Work out the finished part from the listing and answer in its coordinate system (mm). Face numbers are marked on the shaded views. A direction names the side the tool comes from. Coordinates: 2 decimals unless noted, no trailing zeros. Order: outer loops, then holes, each group sorted by start corner. A loop starts at its lowest first (then second) coordinate and runs counter-clockwise, first axis right, second up.
1. Flat-ended cylindrical pins translate along their axes: pin 1 Ø3 at (x, y) = (17.5, -11) entering from +Z; pin 2 Ø6 at (x, z) = (17.5, 7.5) entering from -Y; pin 3 Ø1.1 at (x, z) = (7.5, -3.5) entering from +Y. Find the tip coordinate at first contact, or state that the pin passes through.
2. The part is cut by section C-C, the plane z = 0. Give the vertices of the cut face in (x, y).
3. The part is cut by section D-D, the plane x = 14.5. Give the vertices of the cut face in (y, z).
4. Find the intervals of material crossed by probe 1 along X at (y, z) = (1, 14); probe 2 along Z at (x, y) = (-10, -18); probe 3 along Z at (x, y) = (7.5, -10), in increasing order.
5. The part is cut by section B-B, the plane y = -8. Give the vertices of the cut face in (x, z).
6. Determine the mould class of the marked faces 5, 6 and 7 for opening direction X: +X half, -X half, draft (parallel to the pull), parting line (faces both ways), or undercut.
7. A tool of negligible diameter and unlimited length cuts with its end or side. For the marked faces 1, 2, 3 and 4, from which of +Z, -Z, +X, -X, +Y, -Y can it reach the whole face along a straight path? Write none if from no direction.
8. The part is cut by section A-A, the plane z = -14. Give the vertices of the cut face in (x, y).
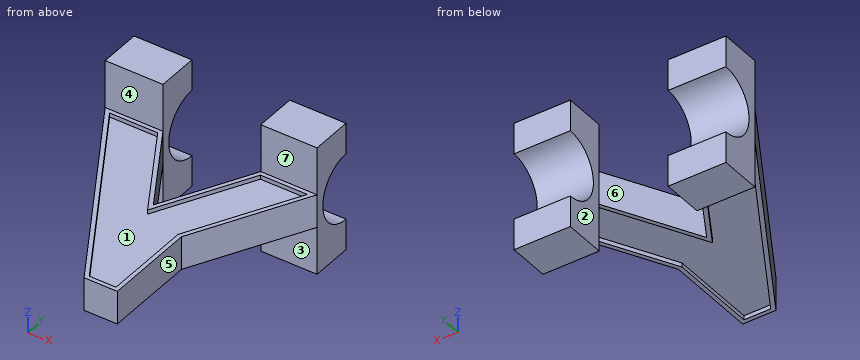
```python
from build123d import *

# Parameters (mm, degrees)
SKETCH_1_W          = 51
SKETCH_1_H          = 31
EXTRUDE_1_DEPTH     = 10
SKETCH_2_R          = 8
CUT_EXTRUDE_1_DEPTH = 51
SKETCH_3_W          = 51
SKETCH_3_H          = 8
EXTRUDE_3_DEPTH     = 49
CUT_EXTRUDE_4_DEPTH = 49
CUT_EXTRUDE_5_DEPTH = 49
CUT_EXTRUDE_6_DEPTH = 1
CUT_EXTRUDE_7_DEPTH = 1


with BuildPart() as part:
    # Эскиз1 → Бобышка-Вытянуть1 (new body)
    with BuildSketch(Plane(origin=(0, 0, 0), x_dir=(1, 0, 0), z_dir=(0, 1, 0))):
        Rectangle(SKETCH_1_W, SKETCH_1_H)
    extrude(amount=EXTRUDE_1_DEPTH)

    # Эскиз2 → Вырез-Вытянуть1 (cut)
    with BuildSketch(Plane(origin=(25.5, 0, 0), x_dir=(0, 0, -1), z_dir=(1, 0, 0))):
        with Locations((0, 10)):
            Circle(SKETCH_2_R)
    extrude(amount=-CUT_EXTRUDE_1_DEPTH, mode=Mode.SUBTRACT)

    # Эскиз3 → Бобышка-Вытянуть3 (add)
    with BuildSketch(Plane.XZ):
        Rectangle(SKETCH_3_W, SKETCH_3_H)
    extrude(amount=EXTRUDE_3_DEPTH)

    # Эскиз4 → Вырез-Вытянуть4 (cut)
    with BuildSketch(Plane(origin=(0, 0, -4), x_dir=(-1, 0, 0), z_dir=(0, 0, -1))):
        Polygon((25.5, -49), (25.5, 0), (-3.5, -49), align=None)
        Polygon((-11.5, -26.802834127), (-25.5, 0), (-25.5, -49), (-11.5, -49), align=None)
        Polygon((11.587587539, 0), (-11.959179604, 0), (-0.863572713, -21.247079042), align=None)
    extrude(amount=-CUT_EXTRUDE_4_DEPTH, mode=Mode.SUBTRACT)

    # Эскиз6 → Вырез-Вытянуть5 (cut)
    with BuildSketch(Plane(origin=(0, 0, 0), x_dir=(-1, 0, 0), z_dir=(0, -1, 0))):
        Polygon((11.587587539, 4), (11.587587539, -15.5), (-11.959179604, -15.5), (-11.959179604, -4), (-11.959179604, 4), (-11.959179604, 15.5), (11.587587539, 15.5), align=None)
    extrude(amount=-CUT_EXTRUDE_5_DEPTH, mode=Mode.SUBTRACT)

    # Эскиз7 → Вырез-Вытянуть6 (cut)
    with BuildSketch(Plane(origin=(0, 0, -4), x_dir=(-1, 0, 0), z_dir=(0, 0, -1))):
        Polygon((23.746151768, -1), (12.160628495, -1), (-0.913951596, -23.310903643), (-12.56510683, -1), (-23.849468801, -1), (-10.5, -26.557399854), (-10.5, -48), (-4.070174763, -48), align=None)
    extrude(amount=-CUT_EXTRUDE_6_DEPTH, mode=Mode.SUBTRACT)

    # Эскиз8 → Вырез-Вытянуть7 (cut)
    with BuildSketch(Plane.XY.offset(4)):
        Polygon((12.56510683, -1), (0.913951596, -23.310903643), (-12.160628495, -1), (-23.746151768, -1), (4.070174763, -48), (10.5, -48), (10.5, -26.557399854), (23.849468801, -1), align=None)
    extrude(amount=-CUT_EXTRUDE_7_DEPTH, mode=Mode.SUBTRACT)


solid = part.part
```
Geometry says:
1. pin 1: stops at z = 4
1. pin 2: stops at y = 0
1. pin 3: stops at y = -7.49
2. outline: (-25.5, 0) - (3.5, -49) - (11.5, -49) - (11.5, -26.8) - (25.5, 0) - (25.5, 2) - (11.96, 2) - (11.96, 0) - (0.86, -21.25) - (-11.59, 0) - (-11.59, 2) - (-25.5, 2) - close
3. outline: (-21.06, -4) - (-18.9, -4) - (-18.9, -3) - (-1, -3) - (-1, -4) - (0, -4) - (0, -15.5) - (10, -15.5) - (10, -8) arc R8 cw to (10, 8) - (10, 15.5) - (0, 15.5) - (0, 4) - (-1, 4) - (-1, 3) - (-18.9, 3) - (-18.9, 4) - (-21.06, 4) - close
4. probe 1: x = -25.5 to -11.59, 11.96 to 25.5
4. probe 2: z = -3 to 3
4. probe 3: z = -4 to 4
5. outline: (-20.77, -4) - (-19.6, -4) - (-19.6, -3) - (-8.06, -3) - (-8.06, -4) - (-6.9, -4) - (-6.9, 4) - (-8.06, 4) - (-8.06, 3) - (-19.6, 3) - (-19.6, 4) - (-20.77, 4) - close; (7.78, -4) - (8.91, -4) - (8.91, -3) - (20.19, -3) - (20.19, -4) - (21.32, -4) - (21.32, 4) - (20.19, 4) - (20.19, 3) - (8.91, 3) - (8.91, 4) - (7.78, 4) - close
6. face 5: +X half
6. face 6: undercut
6. face 7: draft
7. face 1: +Z
7. face 2: +Z, -Z, +Y
7. face 3: -Z, +X, -X, -Y
7. face 4: +Z, +X, -X, -Y
8. outline: (-25.5, 0) - (-11.59, 0) - (-11.59, 10) - (-25.5, 10) - close; (11.96, 0) - (25.5, 0) - (25.5, 10) - (11.96, 10) - close
